from build123d import *

# Parameters (mm, degrees)
ESQUISSE1_W             = 40
ESQUISSE1_H             = 8
BOSS_EXTRU_1_DEPTH      = 8
ESQUISSE2_W             = 20
ESQUISSE2_H             = 8
BOSS_EXTRU_2_DEPTH      = 12
ESQUISSE3_W             = 20
ESQUISSE3_H             = 20
BOSS_EXTRU_3_DEPTH      = 3
CONG_1_R                = 3
ESQUISSE4_R             = 1.6
ENL_V_MAT_EXTRU_1_DEPTH = 47.054315759
ESQUISSE5_R             = 2.1
ENL_V_MAT_EXTRU_2_DEPTH = 47.054315759


with BuildPart() as part:
    # Esquisse1 → Boss.-Extru.1 (new body)
    with BuildSketch(Plane.XY):
        with Locations((20, 4)):
            Rectangle(ESQUISSE1_W, ESQUISSE1_H)
    extrude(amount=BOSS_EXTRU_1_DEPTH)

    # Esquisse2 → Boss.-Extru.2 (add)
    with BuildSketch(Plane.XY.offset(8)):
        with Locations((10, 4)):
            Rectangle(ESQUISSE2_W, ESQUISSE2_H)
    extrude(amount=BOSS_EXTRU_2_DEPTH)

    # Esquisse3 → Boss.-Extru.3 (add)
    with BuildSketch(Plane(origin=(0, 8, 0), x_dir=(1, 0, 0), z_dir=(0, 1, 0))):
        with Locations((10, -10)):
            Rectangle(ESQUISSE3_W, ESQUISSE3_H)
    extrude(amount=BOSS_EXTRU_3_DEPTH)

    # Congé1
    cong_1_edges = [part.edges().sort_by_distance(p)[0] for p in [
        (20, 5.5, 20),
        (40, 4, 8),
        (0, 5.5, 0),
        (0, 5.5, 20),
        (20, 4, 8),
        (20, 8, 4),
    ]]
    fillet(cong_1_edges, radius=CONG_1_R - 0.0001)  # a hair under: the kernel refuses the full size

    # Esquisse4 → Enlèv. mat.-Extru.1 (cut, through all)
    with BuildSketch(Plane(origin=(0, 0, 0), x_dir=(-1, 0, 0), z_dir=(0, 0, -1))):
        with Locations((-30.6, 4)):
            Circle(ESQUISSE4_R)
    extrude(amount=-ENL_V_MAT_EXTRU_1_DEPTH, mode=Mode.SUBTRACT)

    # Esquisse5 → Enlèv. mat.-Extru.2 (cut, through all)
    with BuildSketch(Plane.XZ):
        with Locations(Location((10, 10, 0), (0, 0, 270))):
            Circle(ESQUISSE5_R)
    extrude(amount=-ENL_V_MAT_EXTRU_2_DEPTH, mode=Mode.SUBTRACT)


solid = part.part
Work out the finished part from the listing and answer in its coordinate system (mm). A direction names the side the tool comes from. Coordinates: 2 decimals unless noted, no trailing zeros. Order: outer loops, then holes, each group sorted by start corner. A loop starts at its lowest first (then second) coordinate and runs counter-clockwise, first axis right, second up. Notation, with made-up numbers: (26.5, -27.5) - (79.5, -27.5) arc R23 ccw to (79.5, 4.5) - close; hole circle Ø7 at (71.25, -15). An arc over 180 degrees is marked (long way). Put each result on its own line as item: value. Start each with the question number.
1) For a pull along X with two mould halves and no side action, classify faces 1 (the cylindrical face through (10.09, 5.42, 12.1)), 2 (the cylindrical face through (0.86, 5.58, 19.1)), 3 (the cylindrical face through (20.86, 4.35, 8.9)) as released by +X, released by -X, zero draft, split by the parting line, or undercut.
2) Find section D-D (y = 1.25). Give the vertices of the cut face in (x, z).
3) Find section A-A (y = 4). Give the vertices of the cut face in (x, z), plus the area to 3 significant figures.
4) Find section C-C (z = 11.5). Give the vertices of the cut face in (x, y).
5) Find section B-B (x = 30.6). Give the vertices of the cut face in (y, z).
6) For faces 4 (the flat face through (28, 4, 8)), 5 (the flat face through (40, 4, 2)), 6 (the flat face through (31, 8, 4)), determine the directions among +Z, -Z, +X, -X, +Y, -Y from which every point of the face is accessible in a straight line to the end or side of a thin tool.
7) Find the intervals of material crossed by line 1 (Y direction, x = 30.6, z = 4.25); line 2 (Z direction, x = 35.5, y = 1.5); line 3 (X direction, y = 4.25, z = 10), in increasing order. Write a range as from..to.
8) Flat-ended cylindrical pins translate along their axes: pin 1 (2.5 mm diameter, centred on x = 30.5, y = 5, fed in from +Z); pin 2 (2.5 mm diameter, centred on x = 10, z = 10, fed in from -Y); pin 3 (2.5 mm diameter, centred on x = 32.5, z = 4, fed in from +Y). Find the tip coordinate at first contact, or state that the pin passes through.
Results list:
1. face 1: undercut
1. face 2: released by -X
1. face 3: released by +X
2. outline: (0, 3) arc R3 ccw to (3, 0) - (40, 0) - (40, 5) arc R3 ccw to (37, 8) - (23, 8) arc R3 cw to (20, 11) - (20, 17) arc R3 ccw to (17, 20) - (3, 20) arc R3 ccw to (0, 17) - close; hole circle Ø4.2 at (10, 10)
3. outline: (0, 3) arc R3 ccw to (3, 0) - (29, 0) - (29, 8) - (23, 8) arc R3 cw to (20, 11) - (20, 17) arc R3 ccw to (17, 20) - (3, 20) arc R3 ccw to (0, 17) - close; (32.2, 0) - (40, 0) - (40, 5) arc R3 ccw to (37, 8) - (32.2, 8) - close; hole circle Ø4.2 at (10, 10)
3. area: 515 mm^2
4. outline: (0, 0) - (8.53, 0) - (8.53, 11) - (0, 11) - close; (11.47, 0) - (20, 0) - (20, 11) - (11.47, 11) - close
5. outline: (0, 0) - (2.4, 0) - (2.4, 8) - (0, 8) - close; (5.6, 0) - (8, 0) - (8, 8) - (5.6, 8) - close
6. face 4: +Z, +X, +Y, -Y
6. face 5: +Z, -Z, +X, +Y, -Y
6. face 6: +Z, -Z, +X, +Y
7. line 1: y = 0..2.4, 5.6..8
7. line 2: z = 0..8
7. line 3: x = 0..7.9, 12.1..20.17
8. pin 1: stops at z = 8
8. pin 2: passes through
8. pin 3: stops at y = 8
